The model under review builds one solid part; all positions refer to its coordinate system, in mm. A direction names the side the tool comes from. Round coordinates to 2 decimals unless told otherwise and drop trailing zeros. Order: outer loops, then holes, each group sorted by start corner. A loop starts at its lowest first (then second) coordinate and runs counter-clockwise, first axis right, second up.
1) To check wall thickness, follow L1, parallel to X at y = 45, z = -310; L2, parallel to Z at x = 25, y = 47.75; L3, parallel to Z at x = -5, y = 23.5. State the ranges of each line that lie inside material, in increasing order.
2) Mouldability with a two-part tool opening along Y and no side actions: class faces 5 (the face through (-136.984, 120.747, -9.86)), 6 (the face through (-149.993, 120.66, -9.86)), 7 (the face through (-91, 115, -200)) as pulls with the +Y half, pulls with the -Y half, needs draft (parallel to the pull), parting line crosses it, or undercut.
3) Consider section C-C (y = 129). Give the boundary of the cut face in (x, z), then the cut area to 3 significant figures.
4) Consider section B-B (z = -317). Give the boundary of the cut face in (x, y), then the cut area to 3 significant figures.
5) Consider section D-D (z = -104). Give the boundary of the cut face in (x, y).
6) Clearance check with flat-ended pins moving along their axes: P1, Ø5, axis at x = -2, y = 112, coming from the -Z side; P2, Ø4, axis at y = 50.5, z = -233.5, coming from the +X side; P3, Ø20.5, axis at x = -120, y = 120, coming from the +Z side. State where each tip first meets the part, or that it passes through.
7) Machinability: for faces 1 (the face through (-110, 17, -157)), 2 (the face through (0, 19.7, -107.2)), 3 (the face through (-43.491, 109.656, -9.86)), 4 (the face through (-54, 20, -200)), which of the approach directions +Z, -Z, +X, -X, +Y, -Y give a long, thin tool a straight path to every point of the face, cutting with its end or side? Answer none if there is none.
8) Consider section A-A (y = 170). Give the boundary of the cut face in (x, z).
Autodesk Inventor part; units mm, degrees
ref_plane "YZ Plane" through (0, 0, 0) normal (1, 0, 0) x (0, 1, 0)
ref_plane "XZ Plane" through (0, 0, 0) normal (0, 1, 0) x (-1, 0, 0)
ref_plane "XY Plane" through (0, 0, 0) normal (0, 0, 1) x (1, 0, 0)
sketch "Boceto1" plane through (0, 0, 0) normal (0, 1, 0) x (-1, 0, 0)
  line L0 (0, 0) -> (110, 0)
  line L1 (110, 0) -> (110, -200)
  line L2 (110, -200) -> (0, -200)
  line L3 (0, -200) -> (0, 0)
  circle A0 centre (55, -100) radius 17
  dimension "d0" = 110
  dimension "d1" = 200
extrude "Extrusión1" add sketch "Boceto1" along normal blind 20
sketch "Boceto2" plane through (-110, 0, 0) normal (0, 0, 1) x (1, 0, 0)
  line L0 (110, 20) -> (0, 20)
  line L1 (0, 20) -> (55, 20)
  line L2 (110, 0) -> (0, 0)
  line L3 (110, 20) -> (110, 120)
  circle A0 centre (80, 120) radius 17
  arc A1 (110, 120) -> (80, 150) centre (80, 120) ccw
  circle A2 centre (-10, 120) radius 17
  arc A3 (-10, 150) -> (-10, 90) centre (-10, 120) ccw
  line L4 (-10, 90) -> (55, 90)
  line L5 (55, 90) -> (55, 20)
  line L6 (-10, 150) -> (80, 150)
  dimension "d8" = 55
extrude "Extrusión2" add sketch "Boceto2" against normal blind 20
sketch "Boceto3" plane through (0, 0, -200) normal (0, 0, -1) x (-1, 0, 0)
  line L0 (110, 20) -> (0, 20)
  line L1 (0, 20) -> (0, 60)
  line L2 (0, 60) -> (110, 60)
  line L3 (110, 60) -> (110, 20)
  point P0 (0, 0)
  dimension "d19" = 110
  dimension "d20" = 40
extrude "Extrusión3" add sketch "Boceto3" against normal blind 20
sketch "Boceto4" plane through (0, 0, -200) normal (0, 0, -1) x (-1, 0, 0)
  line L0 (0, 0) -> (110, 0)
  line L1 (110, 0) -> (110, 60)
  circle A0 centre (120, 170) radius 17
  arc A1 (148.016, 159.2713) -> (96, 188) centre (120, 170) ccw
  line L2 (110, 60) -> (148.016, 159.2713)
  line L3 (0, 60) -> (96, 188)
  line L4 (0, 60) -> (110, 60)
  line L5 (0, 60) -> (110, 60)
extrude "Extrusión4" add sketch "Boceto4" against normal blind 20
sketch "Boceto5" plane through (0, 0, 0) normal (1, 0, 0) x (0, 0, -1)
  line L0 (0, 0) -> (200, 0)
  line L1 (200, 0) -> (200, 60)
  line L2 (200, 60) -> (180, 60)
  line L3 (180, 20) -> (180, 60)
  line L4 (20, 20) -> (180, 20)
  line L5 (20, 120) -> (20, 20)
  line L6 (0, 120) -> (20, 120)
  line L7 (0, 0) -> (0, 120)
  line L8 (180, 20) -> (180, 60)
  line L9 (180, 60) -> (310, 60)
  line L10 (310, 60) -> (310, 40)
  line L11 (310, 40) -> (180, 40)
  line L12 (180, 40) -> (180, 60)
  dimension "d30" = 130
  dimension "d31" = 20
extrude "Extrusión5" add sketch "Boceto5" against normal blind 110 contours L11 L3 L2 L1 | L1 L9 L10 L11
sketch "Boceto6" plane through (0, 60, -200) normal (0, 1, 0) x (1, 0, 0)
  line L0 (0, 0) -> (-110, 0)
  line L1 (0, 110) -> (0, 0)
  line L2 (0, 110) -> (-110, 110)
  line L3 (-110, 0) -> (-110, 110)
  line L4 (-96, 0) -> (0, 0)
  line L5 (0, 0) -> (0, 110)
  line L6 (0, 0) -> (0, 50.2087)
  line L7 (0, 110) -> (-70, 110)
  line L8 (0, 110) -> (-110, 110)
  circle A0 centre (-70, 110) radius 17
  arc A1 (-70, 150) -> (-110, 110) centre (-70, 110) ccw
  arc A2 (21.6667, 70.1391) -> (25, 150) centre (25, 110) ccw
  circle A3 centre (25, 110) radius 17
  line L9 (25, 150) -> (-70, 150)
  arc A4 (21.6667, 70.1391) -> (0, 50.2087) centre (20, 50.2087) ccw
  line L10 (-110, 110) -> (-110, 0)
  line L11 (-110, 110) -> (-110, 50.2087)
  line L12 (-110, 50.2087) -> (0, 50.2087)
  point P0 (0, -200)
  point P1 (0, 78.775)
  point P2 (-110, 50.2087)
  point P3 (-87, 110)
  point P4 (-53, 110)
  dimension "d41" = 20
extrude "Extrusión6" add sketch "Boceto6" against normal blind 20 contours L12 L3 L2 A0 L1 | L1 L2 A0 A1 L9 A2 A4
extrude "Extrusión7" cut sketch "Boceto6" against normal blind 20 contours A0 L2 picked at (-58.8313, 108.6439)
properties part number "Pieza4Miniproyecto"
Answer below:
1. L1: x = -110 to -87, -53 to 8, 42 to 65
1. L2: z = -350 to -327, -293 to -270
1. L3: z = -200 to -180, -20 to 0
2. face 5: undercut
2. face 6: parting line crosses it
2. face 7: needs draft
3. outline: (-148.62, -20) - (-134.42, -20) - (-134.42, 0) - (-148.62, 0) - close; (-136.42, -200) - (-51.75, -200) - (-51.75, -180) - (-136.42, -180) - close; (-105.58, -20) - (-44.42, -20) - (-44.42, 0) - (-105.58, 0) - close; (-15.58, -20) - (-1.38, -20) - (-1.38, 0) - (-15.58, 0) - close
3. area: 3,480 mm2
4. outline: (-109.38, 40) - (-85.49, 40) - (-85.49, 60) - (-109.38, 60) - close; (-54.51, 40) - (9.51, 40) - (9.51, 60) - (-54.51, 60) - close; (40.49, 40) - (64.38, 40) - (64.38, 60) - (40.49, 60) - close
4. area: 2,240 mm2
5. outline: (-110, 0) - (-71.52, 0) - (-71.52, 20) - (-110, 20) - close; (-38.48, 0) - (0, 0) - (0, 20) - (-38.48, 20) - close
6. P1: stops at z = -20
6. P2: stops at x = 0
6. P3: stops at z = -180
7. face 1: +Z, -Z, -X, -Y
7. face 2: +Z, +X, +Y, -Y
7. face 3: +Z
7. face 4: -Z, +X, -X, -Y
8. outline: (-150, -200) - (-137, -200) - (-137, -180) - (-150, -180) - close; (-103, -200) - (-82.5, -200) - (-82.5, -180) - (-103, -180) - close
